```python
from build123d import *

# Parameters (mm, degrees)
BOSS_EXTRUDE1_DEPTH = 5
SKETCH2_R           = 2.1
CUT_EXTRUDE1_DEPTH  = 10
SKETCH3_R           = 10
BOSS_EXTRUDE2_DEPTH = 1
SKETCH4_R           = 2.75
BOSS_EXTRUDE3_DEPTH = 5
SKETCH5_W           = 50
SKETCH5_H           = 30
SKETCH5_W_2         = 30
SKETCH5_H_2         = 10
CUT_EXTRUDE2_DEPTH  = 52.14684741
BOSS_EXTRUDE4_START = 1
BOSS_EXTRUDE4_DEPTH = 1


with BuildPart() as part:
    # Sketch1 → Boss-Extrude1 (new, symmetric)
    with BuildSketch(Plane.XY):
        Polygon((15, 5), (15, 0), (0, 0), (0, 19), (15, 19), (15, 14), (20, 14), (20, 24), (-10, 24), (-10, -5), (20, -5), (20, 5), align=None)
    extrude(amount=BOSS_EXTRUDE1_DEPTH, both=True)

    # Sketch2 → Cut-Extrude1 (cut)
    with BuildSketch(Plane.ZY.offset(10)):
        with Locations(Location((0, 9.5, 0), (0, 0, 270))):
            Circle(SKETCH2_R)
    extrude(amount=-CUT_EXTRUDE1_DEPTH, mode=Mode.SUBTRACT)

    # Sketch3 → Boss-Extrude2 (add)
    with BuildSketch(Plane(origin=(0, 24, 0), x_dir=(1, 0, 0), z_dir=(0, 1, 0))):
        with Locations(Location((0, 0, 0), (0, 0, 180))):
            Circle(SKETCH3_R)
    extrude(amount=BOSS_EXTRUDE2_DEPTH)

    # Sketch4 → Boss-Extrude3 (add)
    with BuildSketch(Plane.XY):
        with BuildLine():
            Line((10, 25), (-10, 25))
            Line((-10, 25), (-4.615384615, 37.923076923))
            ThreePointArc((-4.615384615, 37.923076923), (0, 41), (4.615384615, 37.923076923))
            Line((4.615384615, 37.923076923), (10, 25))
        make_face()
        with Locations((0, 36)):
            Circle(SKETCH4_R, mode=Mode.SUBTRACT)
    extrude(amount=BOSS_EXTRUDE3_DEPTH)

    # Sketch5 → Cut-Extrude2 (cut, through all)
    with BuildSketch(Plane.XZ.offset(5)):
        with Locations((5, 0)):
            Rectangle(SKETCH5_W, SKETCH5_H)
        with Locations((5, 0)):
            Rectangle(SKETCH5_W_2, SKETCH5_H_2, mode=Mode.SUBTRACT)
    extrude(amount=-CUT_EXTRUDE2_DEPTH, mode=Mode.SUBTRACT)

    # Sketch6 → Boss-Extrude4 (add)
    with BuildSketch(Plane.XZ.offset(-25).offset(BOSS_EXTRUDE4_START)):
        with BuildLine():
            Line((10, 5), (8.660254038, 5))
            ThreePointArc((8.660254038, 5), (9.659258263, 2.588190451), (10, 0))
            Line((10, 0), (10, 5))
        make_face()
        with BuildLine():
            Line((-10, 5), (-10, 0))
            ThreePointArc((-10, 0), (-9.659258263, 2.588190451), (-8.660254038, 5))
            Line((-8.660254038, 5), (-10, 5))
        make_face()
    extrude(amount=-BOSS_EXTRUDE4_DEPTH)


solid = part.part
```
Work out the finished part from the listing and answer in its coordinate system (mm). A direction names the side the tool comes from. Coordinates: 2 decimals unless noted, no trailing zeros. Loops run counter-clockwise (first coordinate to the right, second up) from the corner with the lowest first, then second, coordinate; pieces in that order, holes last. Notation, with made-up numbers: (6.5, 45) - (37.5, 45) arc R14 ccw to (37.5, 66) - close; hole circle Ø3 at (81, 79.5). An arc over 180 degrees is marked (long way). Use a Markdown table: item, result.
Item 1: Find section C-C, the plane x = -0.5. Determine the outline of the cut face in (y, z).
Evaluation:
| item | result |
|---|---|
| outline | (-5, -5) - (25, -5) - (25, 0) - (33.3, 0) - (33.3, 5) - (-5, 5) - close; (38.7, 0) - (40.97, 0) - (40.97, 5) - (38.7, 5) - close; hole circle Ø4.2 at (9.5, 0) |
Item 2: The mould has two halves that part along X. Classify faces 1 (the flat face through (0, 7, 0)), 2 (the flat face through (-7.345, 31.371, 2.465)), 3 (the flat face through (-1, 13, 5)): +X half, -X half, draft (parallel to the pull), parting line (faces both ways), or undercut.
Evaluation:
| item | result |
|---|---|
| face 1 | undercut |
| face 2 | -X half |
| face 3 | draft |
Item 3: For faces 4 (the flat face through (-9.5, 24, -3.8)), 5 (the flat face through (15, 17, 0)), 6 (the flat face through (0, 31, 0)), 7 (the flat face through (10, 24.5, 2.5)), determine the directions among +Z, -Z, +X, -X, +Y, -Y from which every point of the face is accessible in a straight line to the end or side of a thin tool.
Evaluation:
| item | result |
|---|---|
| face 4 | -Z, -X, +Y |
| face 5 | +Z, -Z |
| face 6 | -Z, +X, -X, +Y |
| face 7 | +Z, -Z, +X, +Y |
Item 4: Find section A-A, the plane x = 18. Determine the outline of the cut face in (y, z), and give its area (3 significant figures).
Evaluation:
| item | result |
|---|---|
| outline | (-5, -5) - (5, -5) - (5, 5) - (-5, 5) - close; (14, -5) - (24, -5) - (24, 5) - (14, 5) - close |
| area | 200 mm2 |
Item 5: Given pin 1 Ø0.8 at (y, z) = (24.5, 1.5) entering from +X; pin 2 Ø5 at (x, z) = (8, 2) entering from +Y; pin 3 Ø5.5 at (x, z) = (-0.5, -3.5) entering from +Y, each flat-ended and moving along its own axis, determine where each tip first touches the part or whether it passes through.
Evaluation:
| item | result |
|---|---|
| pin 1 | stops at x = 10 |
| pin 2 | stops at y = 35.8 |
| pin 3 | stops at y = 25 |
Item 6: Find section B-B, the plane y = 2. Determine the outline of the cut face in (x, z), and give its area (3 significant figures).
Evaluation:
| item | result |
|---|---|
| outline | (-10, -5) - (0, -5) - (0, 5) - (-10, 5) - close; (15, -5) - (20, -5) - (20, 5) - (15, 5) - close |
| area | 150 mm2 |
Item 7: Consider probe 1 along X at (y, z) = (17.5, 0.75); probe 2 along Z at (x, y) = (-4.5, 9.5); probe 3 along Y at (x, z) = (14.25, -3.5). Determine where each line is inside the solid, lowest interval first. Write a range as from..to.
Evaluation:
| item | result |
|---|---|
| probe 1 | x = -10..0, 15..20 |
| probe 2 | z = -5..-2.1, 2.1..5 |
| probe 3 | y = -5..0, 19..24 |
